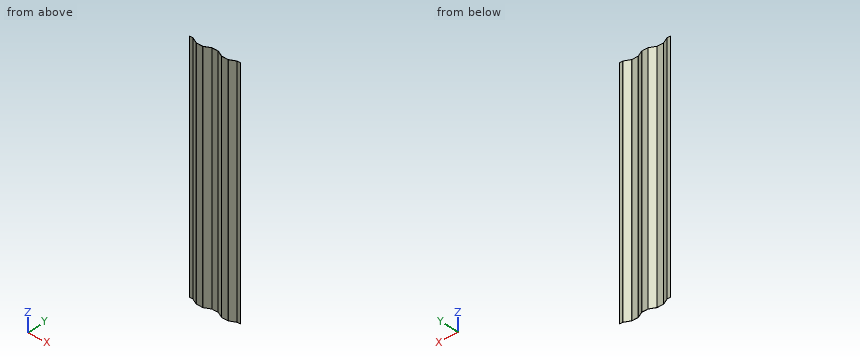
from build123d import *

# Parameters (mm, degrees)
F1_DEPTH = 2629
F2_W     = 721.211998
F2_H     = 2677.757788
F3_DEPTH = 36.001


with BuildPart() as f1:
    # F0 (on Top) → F1 (new body)
    with BuildSketch(Plane.XY):
        with BuildLine():
            ThreePointArc((103.213446, 15.932448), (104.661294, 15.401879), (106.192738, 15.221745))
            Line((106.192738, 15.221745), (175.807262, 15.221745))
            ThreePointArc((175.807262, 15.221745), (177.338706, 15.401879), (178.786554, 15.932448))
            Line((178.786554, 15.932448), (245.381676, 49.621745))
            Line((245.381676, 49.621745), (314.618324, 49.621745))
            Line((314.618324, 49.621745), (381.213446, 15.932448))
            ThreePointArc((381.213446, 15.932448), (382.661294, 15.401879), (384.192738, 15.221745))
            Line((384.192738, 15.221745), (453.807262, 15.221745))
            ThreePointArc((453.807262, 15.221745), (455.338706, 15.401879), (456.786554, 15.932448))
            Line((456.786554, 15.932448), (523.381676, 49.621745))
            Line((523.381676, 49.621745), (592.618324, 49.621745))
            Line((592.618324, 49.621745), (659.213446, 15.932448))
            ThreePointArc((659.213446, 15.932448), (660.661294, 15.401879), (662.192738, 15.221745))
            Line((662.192738, 15.221745), (731.807262, 15.221745))
            ThreePointArc((731.807262, 15.221745), (733.338706, 15.401879), (734.786554, 15.932448))
            Line((734.786554, 15.932448), (801.381676, 49.621745))
            Line((801.381676, 49.621745), (870.618324, 49.621745))
            Line((870.618324, 49.621745), (937.213446, 15.932448))
            ThreePointArc((937.213446, 15.932448), (938.661294, 15.401879), (940.192738, 15.221745))
            Line((940.192738, 15.221745), (1009.807262, 15.221745))
            ThreePointArc((1009.807262, 15.221745), (1011.338706, 15.401879), (1012.786554, 15.932448))
            Line((1012.786554, 15.932448), (1079.381676, 49.621745))
            Line((1079.381676, 49.621745), (1116, 49.621745))
            Line((1116, 49.621745), (1116, 51.221745))
            Line((1116, 51.221745), (1080.192738, 51.221745))
            ThreePointArc((1080.192738, 51.221745), (1079.032553, 51.08528), (1077.935699, 50.683334))
            Line((1077.935699, 50.683334), (1012.064301, 17.360156))
            ThreePointArc((1012.064301, 17.360156), (1010.967447, 16.95821), (1009.807262, 16.821745))
            Line((1009.807262, 16.821745), (940.192738, 16.821745))
            ThreePointArc((940.192738, 16.821745), (939.032553, 16.95821), (937.935699, 17.360156))
            Line((937.935699, 17.360156), (872.064301, 50.683334))
            ThreePointArc((872.064301, 50.683334), (870.967447, 51.08528), (869.807262, 51.221745))
            Line((869.807262, 51.221745), (802.192738, 51.221745))
            ThreePointArc((802.192738, 51.221745), (801.032553, 51.08528), (799.935699, 50.683334))
            Line((799.935699, 50.683334), (734.064301, 17.360156))
            ThreePointArc((734.064301, 17.360156), (732.967447, 16.95821), (731.807262, 16.821745))
            Line((731.807262, 16.821745), (662.192738, 16.821745))
            ThreePointArc((662.192738, 16.821745), (661.032553, 16.95821), (659.935699, 17.360156))
            Line((659.935699, 17.360156), (594.064301, 50.683334))
            ThreePointArc((594.064301, 50.683334), (592.967447, 51.08528), (591.807262, 51.221745))
            Line((591.807262, 51.221745), (524.192738, 51.221745))
            ThreePointArc((524.192738, 51.221745), (523.032553, 51.08528), (521.935699, 50.683334))
            Line((521.935699, 50.683334), (456.064301, 17.360156))
            ThreePointArc((456.064301, 17.360156), (454.967447, 16.95821), (453.807262, 16.821745))
            Line((453.807262, 16.821745), (384.192738, 16.821745))
            ThreePointArc((384.192738, 16.821745), (383.032553, 16.95821), (381.935699, 17.360156))
            Line((381.935699, 17.360156), (316.064301, 50.683334))
            ThreePointArc((316.064301, 50.683334), (314.967447, 51.08528), (313.807262, 51.221745))
            Line((313.807262, 51.221745), (246.192738, 51.221745))
            ThreePointArc((246.192738, 51.221745), (245.032553, 51.08528), (243.935699, 50.683334))
            Line((243.935699, 50.683334), (178.064301, 17.360156))
            ThreePointArc((178.064301, 17.360156), (176.967447, 16.95821), (175.807262, 16.821745))
            Line((175.807262, 16.821745), (106.192738, 16.821745))
            ThreePointArc((106.192738, 16.821745), (105.032553, 16.95821), (103.935699, 17.360156))
            Line((103.935699, 17.360156), (38.064301, 50.683334))
            ThreePointArc((38.064301, 50.683334), (36.967447, 51.08528), (35.807262, 51.221745))
            Line((35.807262, 51.221745), (0, 51.221745))
            Line((0, 51.221745), (0, 49.621745))
            Line((0, 49.621745), (36.618324, 49.621745))
            Line((36.618324, 49.621745), (103.213446, 15.932448))
        make_face()
    extrude(amount=F1_DEPTH)

    # F2 (on face) → F3 (cut, through all)
    with BuildSketch(Plane(origin=(0, 51.221745, 0), x_dir=(-1, 0, 0), z_dir=(0, 1, 0))):
        with Locations((-918.605999, 1290.121106)):
            Rectangle(F2_W, F2_H)
    extrude(amount=-F3_DEPTH, mode=Mode.SUBTRACT)


solid = f1.part
Read the model definition and answer for the solid it produces. Units are mm, in the model's axes. Coordinates: 2 decimals unless noted, no trailing zeros. Order: outer loops, then holes, each group sorted by start corner. A loop starts at its lowest first (then second) coordinate and runs counter-clockwise, first axis right, second up. Notation, with made-up numbers: (53, -2) - (108, -2) arc R30 ccw to (108, 21) - close; hole circle Ø4 at (38.5, 25.5). An arc over 180 degrees is marked (long way). Use one line per item in the form item = value.
(1) Given pin 1 Ø10 at (x, z) = (492.5, 447.5) entering from +Y; pin 2 Ø4 at (y, z) = (42.5, 789.5) entering from -X; pin 3 Ø5 at (x, z) = (120, 404.5) entering from +Y, each flat-ended and moving along its own axis, determine where each tip first touches the part or whether it passes through.
Computed values:
pin_1 = 38.32
pin_2 = 46.74
pin_3 = 16.82
(2) Section A-A, the plane y = 42.5 is taken. Give the vertices of the cut face in (x, z), then the cut area to 3 significant figures.
Computed values:
outline = (50.7, 0) - (54.24, 0) - (54.24, 2629) - (50.7, 2629) - close; (227.76, 0) - (231.3, 0) - (231.3, 2629) - (227.76, 2629) - close; (328.7, 0) - (332.24, 0) - (332.24, 2629) - (328.7, 2629) - close; (505.76, 0) - (509.3, 0) - (509.3, 2629) - (505.76, 2629) - close
area = 37,300 mm²
(3) Section C-C, the plane x = 484 is taken. Give the vertices of the cut face in (y, z), then the cut area to 3 significant figures.
Computed values:
outline = (29.7, 0) - (31.49, 0) - (31.49, 2629) - (29.7, 2629) - close
area = 4,710 mm²
(4) Straight lines are drawn through the part: L1, parallel to X at y = 31, z = 163; L2, parallel to X at y = 28, z = 1184; L3, parallel to X at y = 50, z = 2032.5. For each, find the intervals that lie inside material, in ascending order.
Computed values:
L1 = 73.43 to 76.97, 205.03 to 208.57, 351.43 to 354.97, 483.03 to 486.57
L2 = 79.36 to 82.9, 199.1 to 202.64, 357.36 to 360.9, 477.1 to 480.64
L3 = 0 to 39.42, 242.58 to 317.42, 520.58 to 558
